Part model, mm, in its own coordinate system. A direction names the side the tool comes from. Round coordinates to 2 decimals unless told otherwise and drop trailing zeros. Order: outer loops, then holes, each group sorted by start corner. A loop starts at its lowest first (then second) coordinate and runs counter-clockwise, first axis right, second up. Notation, with made-up numbers: (-13.5, 89) - (6.5, 89) arc R16 cw to (6.5, 114) - close; hole circle Ø4 at (56, 3.5). An arc over 180 degrees is marked (long way). Answer as a JSON object with one key per item and string values.
```python
from build123d import *

# Parameters (mm, degrees)
SKETCH1_R         = 9.525
SKETCH1_R_2       = 8.636
EXTRUDE1_DEPTH    = 457.2
SKETCH2_R         = 34.671
SKETCH2_R_2       = 8.636
EXTRUDE2_DEPTH    = 12.7
SKETCH3_R         = 3.3655
EXTRUDE3_DEPTH    = 458.2
CIRPATTERN1_COUNT = 6
SKETCH4_R         = 10.31875
SKETCH4_R_2       = 8.636
EXTRUDE4_DEPTH    = 3.175


with BuildPart() as part:
    # Sketch1 → Extrude1 (new body)
    with BuildSketch(Plane(origin=(0, 0, 0), x_dir=(1, 0, 0), z_dir=(0, 1, 0))):
        Circle(SKETCH1_R)
        Circle(SKETCH1_R_2, mode=Mode.SUBTRACT)
    extrude(amount=EXTRUDE1_DEPTH)

    # Sketch2 → Extrude2 (add)
    with BuildSketch(Plane(origin=(0, 457.2, 0), x_dir=(1, 0, 0), z_dir=(0, 1, 0))):
        Circle(SKETCH2_R)
        Circle(SKETCH2_R_2, mode=Mode.SUBTRACT)
    extrude(amount=-EXTRUDE2_DEPTH)

    # Sketch3 → Extrude3 (cut, through all)
    with BuildSketch(Plane(origin=(0, 457.2, 0), x_dir=(1, 0, 0), z_dir=(0, 1, 0))):
        with Locations((0, 29.3624)):
            Circle(SKETCH3_R)
    extrude3 = extrude(amount=-EXTRUDE3_DEPTH, mode=Mode.SUBTRACT)

    # CirPattern1: Extrude3 ×6 about axis
    cirpattern1_axis = Axis((0, 0, 0), (0, 1, 0))
    for i in range(1, CIRPATTERN1_COUNT):
        add(extrude3.rotate(cirpattern1_axis, i * 360 / CIRPATTERN1_COUNT), mode=Mode.SUBTRACT)

    # Sketch4 → Extrude4 (add)
    with BuildSketch(Plane.XZ):
        Circle(SKETCH4_R)
        Circle(SKETCH4_R_2, mode=Mode.SUBTRACT)
    extrude(amount=-EXTRUDE4_DEPTH)


solid = part.part
```
Item 1: Cut at A-A (z = 0). Write the cut outline in (x, y) (3 decimals).
Taken from the geometry:
{"outline": "(-34.671, 444.5) - (-9.525, 444.5) - (-9.525, 3.175) - (-10.319, 3.175) - (-10.319, 0) - (-8.636, 0) - (-8.636, 457.2) - (-34.671, 457.2) - close; (8.636, 0) - (10.319, 0) - (10.319, 3.175) - (9.525, 3.175) - (9.525, 444.5) - (34.671, 444.5) - (34.671, 457.2) - (8.636, 457.2) - close"}
Item 2: Cut at B-B (y = 75). Write the cut outline in (x, z) (3 decimals).
Taken from the geometry:
{"outline": "circle Ø19.05 at (0, 0); hole circle Ø17.272 at (0, 0)"}
Item 3: Probe L1, parallel to Z at x = 0, y = 452; L2, parallel to Z at x = 0, y = 298 (3 decimals); L3, parallel to Y at x = -14.5, z = -17. List the from-to ranges inside material, lowest first. Write a range as from..to.
Taken from the geometry:
{"L1": "-34.67..-32.73, -26..-8.64, 8.64..26, 32.73..34.67", "L2": "-9.525..-8.636, 8.636..9.525", "L3": "444.5..457.2"}
Item 4: Two-plate mould, pull along Y, no slides. Class faces 4 (the flat face through (7, 3.175, -7)), 5 (the cylindrical face through (-34.637, 450.939, -1.524)), 6 (the flat face through (5, 0, -8)): pulls with the +Y half, pulls with the -Y half, needs draft (parallel to the pull), parting line crosses it, or undercut.
Taken from the geometry:
{"face 4": "undercut", "face 5": "needs draft", "face 6": "pulls with the -Y half"}
Item 5: Cut at C-C (x = 14.5). Write the cut outline in (y, z).
Taken from the geometry:
{"outline": "(444.5, -31.49) - (457.2, -31.49) - (457.2, 31.49) - (444.5, 31.49) - close"}
Item 6: Drop flat-ended pins along their axis: P1, Ø4, axis at y = 94, z = 13, coming from the -X side; P2, Ø1, axis at x = -9.5, z = 6, coming from the -Y side; P3, Ø5, axis at y = 361, z = 4, coming from the -X side. Give the stop position or say it passes through.
Taken from the geometry:
{"P1": "through", "P2": "y = 444.5", "P3": "x = -9.41"}
Item 7: Tool access for faces 1 (the cylindrical face through (-1.124, 225.4, -8.563)), 2 (the cylindrical face through (-7.559, 220.748, 5.796)), 3 (the cylindrical face through (-2.237, 1.565, -10.073)): list every direction of +Z, -Z, +X, -X, +Y, -Y with a clear straight run to the whole face (end or side of a thin tool).
Taken from the geometry:
{"face 1": "+Y, -Y", "face 2": "none", "face 3": "-Y"}
